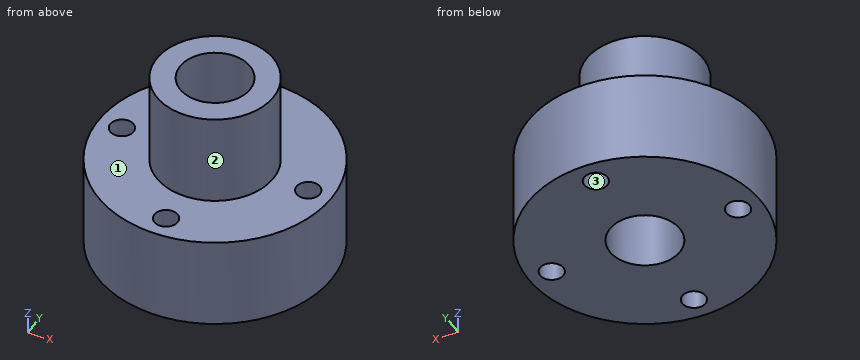
from build123d import *

# Parameters (mm, degrees)
F0_R     = 15.875
F1_DEPTH = 12.7
F2_R     = 7.9375
F3_DEPTH = 25.4
F4_R     = 4.7625
F5_DEPTH = 25.4
F6_R     = 1.5875
F7_DEPTH = 12.7


with BuildPart() as f1:
    # F0 (on Top) → F1 (new body)
    with BuildSketch(Plane.XY):
        Circle(F0_R)
    extrude(amount=F1_DEPTH)

    # F2 (on Top) → F3 (join)
    with BuildSketch(Plane.XY):
        Circle(F2_R)
    extrude(amount=F3_DEPTH)

    # F4 (on Top) → F5 (cut)
    with BuildSketch(Plane.XY):
        Circle(F4_R)
    extrude(amount=F5_DEPTH, mode=Mode.SUBTRACT)

    # F6 (on Top) → F7 (cut)
    with BuildSketch(Plane.XY):
        with Locations((0, 12.7)):
            Circle(F6_R)
        with Locations((12.7, 0)):
            Circle(F6_R)
        with Locations((-12.7, 0)):
            Circle(F6_R)
        with Locations((0, -12.7)):
            Circle(F6_R)
    extrude(amount=F7_DEPTH, mode=Mode.SUBTRACT)


solid = f1.part
The model under review builds one solid part; all positions refer to its coordinate system, in mm. Face numbers are marked on the shaded views. Coordinates: 2 decimals unless noted, no trailing zeros. Write each loop counter-clockwise with the first axis right and the second up, starting at its lowest first coordinate (ties: lowest second). Pieces come first, ordered by that corner, then holes. Notation, with made-up numbers: (61.25, 62.25) - (116.25, 62.25) arc R11 cw to (116.25, 81.25) - close; hole circle Ø2 at (11, -15.75). An arc over 180 degrees is marked (long way). Answer as CSV lines item,"result".
(1) Clearance check with flat-ended pins moving along their axes: pin 1 Ø8 at (x, z) = (1.5, 6) entering from +Y (3 decimals); pin 2 Ø3 at (x, z) = (-11, 10.5) entering from +Y; pin 3 Ø1.5 at (y, z) = (9, 9.5) entering from +X; pin 4 Ø1.5 at (x, z) = (3, 22) entering from +Y. State where each tip first meets the part, or that it passes through.
Data:
pin 1,"stops at y = 15.875"
pin 2,"stops at y = 12.72"
pin 3,"stops at x = 13.56"
pin 4,"stops at y = 7.61"
(2) For line 1 along Y through (x, z) = (0, 10) (1 decimal); line 2 along Z through (x, y) = (-4, -13.5); line 3 along Y through (x, z) = (3, 19), list the stretches that pass through material, from the lowest coordinate up. Write a range as [from, to].
Data:
line 1,"y = [-15.9, -14.3], [-11.1, -4.8], [4.8, 11.1], [14.3, 15.9]"
line 2,"z = [0, 12.7]"
line 3,"y = [-7.35, -3.7], [3.7, 7.35]"
(3) We need section A-A (y = 0). Give the boundary of the cut face in (x, z) (1 decimal), plus the area to 3 significant figures.
Data:
outline,"(-15.9, 0) - (-14.3, 0) - (-14.3, 12.7) - (-15.9, 12.7) - close; (-11.1, 0) - (-4.8, 0) - (-4.8, 25.4) - (-7.9, 25.4) - (-7.9, 12.7) - (-11.1, 12.7) - close; (4.8, 0) - (11.1, 0) - (11.1, 12.7) - (7.9, 12.7) - (7.9, 25.4) - (4.8, 25.4) - close; (14.3, 0) - (15.9, 0) - (15.9, 12.7) - (14.3, 12.7) - close"
area,"282 mm2"
(4) We need section C-C (x = -12.7). Give the boundary of the cut face in (y, z) (1 decimal), plus the area to 3 significant figures.
Data:
outline,"(-9.5, 0) - (-1.6, 0) - (-1.6, 12.7) - (-9.5, 12.7) - close; (1.6, 0) - (9.5, 0) - (9.5, 12.7) - (1.6, 12.7) - close"
area,"202 mm2"
(5) Mouldability with a two-part tool opening along Y and no side actions: class the marked faces 1, 2 and 3 as pulls with the +Y half, pulls with the -Y half, needs draft (parallel to the pull), parting line crosses it, or undercut.
Data:
face 1,"needs draft"
face 2,"parting line crosses it"
face 3,"undercut"
(6) We need section D-D (z = 7). Count the separate pieces of the cut face and the enclosed holes in it, plus the area to 3 significant figures.
Data:
separate pieces,"1"
enclosed holes,"5"
area,"689 mm2"
